Could you check a few things on this model? Use its own coordinates, in mm. A direction names the side the tool comes from. Give positions to 0.01 mm unless a question says otherwise; leave off trailing zeros. Write each loop counter-clockwise with the first axis right and the second up, starting at its lowest first coordinate (ties: lowest second). Pieces come first, ordered by that corner, then holes. Notation, with made-up numbers: M 79.25,78.25 L 130.25,78.25 A13 ccw 130.25,99.25 Z; hole C -14,84 d2. An arc over 180 degrees is marked long. One line per item, written item: value.
Autodesk Inventor part; units mm, degrees
ref_plane "YZ Plane" through (0, 0, 0) normal (1, 0, 0) x (0, 1, 0)
ref_plane "XZ Plane" through (0, 0, 0) normal (0, 1, 0) x (-1, 0, 0)
ref_plane "XY Plane" through (0, 0, 0) normal (0, 0, 1) x (1, 0, 0)
sketch "Sketch1" plane through (0, 0, 0) normal (0, 0, 1) x (1, 0, 0)
  arc A0 (0, 34.29) -> (0, -34.29) centre (0, 0) ccw
  arc A1 (0, 39.37) -> (0, -39.37) centre (0, 0) ccw
  line L0 (0, 0) -> (656.8948, 0)
  arc A2 (656.8948, -34.29) -> (656.8948, 34.29) centre (656.8948, 0) ccw
  arc A3 (656.8948, -39.37) -> (656.8948, 39.37) centre (656.8948, 0) ccw
  line L1 (0, 39.37) -> (656.8948, 39.37)
  line L2 (656.8948, 34.29) -> (0, 34.29)
  line L3 (0, -34.29) -> (656.8948, -34.29)
  line L4 (656.8948, -39.37) -> (0, -39.37)
  dimension "d0" = 68.58
  dimension "d1" = 78.74
  dimension "d2" = 656.8948
  dimension "d3" = 68.58
  dimension "d4" = 78.74
extrude "Extrusion1" add sketch "Sketch1" along normal blind 457.2
properties part number "bult"
1) If we section it at A-A, the plane x = 428: Write out the boundary of the cut face in (y, z), then the cut area to 3 significant figures.
Outcome:
outline: M -39.37,0 L -34.29,0 L -34.29,457.2 L -39.37,457.2 Z; M 34.29,0 L 39.37,0 L 39.37,457.2 L 34.29,457.2 Z
area: 4,650 mm^2
2) If we section it at B-B, the plane y = 0: Write out the boundary of the cut face in (x, z), then the cut area to 3 significant figures.
Outcome:
outline: M -39.37,0 L -34.29,0 L -34.29,457.2 L -39.37,457.2 Z; M 691.18,0 L 696.26,0 L 696.26,457.2 L 691.18,457.2 Z
area: 4,650 mm^2
3) I'm going to push flat-ended pins straight in: pin 1 (8 mm diameter, centred on y = -5.5, z = 389.5, fed in from +X); pin 2 (6 mm diameter, centred on y = -8, z = 65, fed in from +X); pin 3 (8 mm diameter, centred on y = 6.5, z = 81.5, fed in from -X). Where does each tip first touch, or does it pass through?
Outcome:
pin 1: stops at x = 696.24
pin 2: stops at x = 695.95
pin 3: stops at x = -39.29
4) On a 3-axis mill with a long thin cutter (end or side, diameter ignored), from which of +Z, -Z, +X, -X, +Y, -Y can I reach the whole of each face in a straight line? I mean faces 1 (the face through (691.177, 0.754, 225.4)), 2 (the face through (324, 39.37, 225)). Say none if no direction works.
Outcome:
face 1: +Z, -Z
face 2: +Z, -Z, +X, -X, +Y
5) We'd pull the mould along X, two halves only. Please class faces 3 (the face through (696.255, 0.866, 225.4)), 4 (the face through (-34.28, -0.75, 225.4)), 5 (the face through (327, 35, 0)): pulls with the +X half, pulls with the -X half, needs draft (parallel to the pull), parting line crosses it, or undercut.
Outcome:
face 3: pulls with the +X half
face 4: undercut
face 5: needs draft
6) If we section it at C-C, the plane z = 150.5: Write out the boundary of the cut face in (x, y), then the cut area to 3 significant figures.
Outcome:
outline: M 0,-39.37 L 656.89,-39.37 A39.37 ccw 656.89,39.37 L 0,39.37 A39.37 ccw Z; hole M 0,-34.29 L 656.89,-34.29 A34.29 ccw 656.89,34.29 L 0,34.29 A34.29 ccw Z
area: 7,850 mm^2
7) Please list where these lines run through material, in increasing order: L1, parallel to Y at x = 413, z = 167; L2, parallel to X at y = -11, z = 408.5; L3, parallel to X at y = -9, z = 161.5. Write a range as from..to.
Outcome:
L1: y = -39.37..-34.29, 34.29..39.37
L2: x = -37.8..-32.48, 689.37..694.7
L3: x = -38.33..-33.09, 689.98..695.22
